from build123d import *

# Parameters (mm, degrees)
CYLINDER_R        = 1.3
CYLINDER_DEPTH    = 8
CYLINDER001_R     = 1.3
CYLINDER001_DEPTH = 8
EXTRUDE_DEPTH     = 15
CHAMFER_SIZE      = 2


with BuildPart() as cylinder000:
    # Cylinder → Cylinder (new body)
    with BuildSketch(Plane(origin=(12.5, -7.5, 0), x_dir=(1, 0, 0), z_dir=(0, 0, 1))):
        Circle(CYLINDER_R)
    extrude(amount=CYLINDER_DEPTH)


with BuildPart() as fusion:
    # Cylinder001 → Cylinder001 (new body)
    with BuildSketch(Plane(origin=(12.5, -7.5, 36), x_dir=(1, 0, 0), z_dir=(0, 0, 1))):
        Circle(CYLINDER001_R)
    extrude(amount=CYLINDER001_DEPTH)

    # Fusion: union Cylinder000
    add(cylinder000.part)


with BuildPart() as cut:
    # Sketch → Extrude (new body)
    with BuildSketch(Plane.XZ):
        Polygon((0, 0), (25, 0), (10, 15), (10, 29), (25, 44), (0, 44), align=None)
    extrude(amount=EXTRUDE_DEPTH)

    # Chamfer
    chamfer_edges = [cut.edges().sort_by_distance(p)[0] for p in [
        (0, 0, 22),
        (0, -15, 22),
        (17.5, 0, 7.5),
        (17.5, -15, 7.5),
        (10, 0, 22),
        (10, -15, 22),
        (17.5, 0, 36.5),
        (17.5, -15, 36.5),
    ]]
    chamfer(chamfer_edges, length=CHAMFER_SIZE)

    # Cut: cut Fusion
    add(fusion.part, mode=Mode.SUBTRACT)


solid = cut.part
Check sheet for the modelled part. Datum: model origin and axes. Units: mm. A direction names the side the tool comes from. Round coordinates to 2 decimals unless told otherwise and drop trailing zeros. Order: outer loops, then holes, each group sorted by start corner. A loop starts at its lowest first (then second) coordinate and runs counter-clockwise, first axis right, second up. Notation, with made-up numbers: M 36.25,23 L 67.25,23 A25 ccw 67.25,62 Z; hole C -26.75,2 d6. An arc over 180 degrees is marked long. One line per item, written item: value. Start each with the question number.
1. Section check C-C on y = -7.5. Enter the section's corners in (x, z), and give its area (3 significant figures).
2. Access from +Z, -Z, +X, -X, +Y, -Y to the whole of each face (thin tool, end or side, straight path). Record for faces 5 (the flat face through (18, -7, 7)), 6 (the flat face through (9, -1, 22)), 7 (the cylindrical face through (12.22, -8.77, 3.94)), 8 (the flat face through (16.381, -14.014, 36.815)), 9 (the cylindrical face through (12.22, -8.77, 39.94)).
3. Release check for a two-part mould opening along Z. For faces 1 (the flat face through (16.6, -0.99, 6.97)), 2 (the flat face through (16.381, -0.986, 36.815)), 3 (the flat face through (12, -7, 36)), 4 (the flat face through (1, -1, 22)) record: released by +Z, released by -Z, zero draft, split by the parting line, or undercut.
4. Section check A-A on x = 12.5. Enter the section's corners in (y, z).
5. Section check B-B on z = 21. Enter the section's corners in (x, y), and give its area (3 significant figures).
6. Scan lines: line 1 along Y through (x, z) = (12.5, 39.25); line 2 along Z through (x, y) = (17, -10.25); line 3 along Z through (x, y) = (18.5, -10.5). Record each from-to range of solid material in increasing order.
7. Section check D-D on z = 7. Enter the section's corners in (x, y).
8. Gauge pin test, flat ends, axial feed: P1, Ø9, axis at y = -8, z = 21.5, coming from the +X side; P2, Ø2, axis at x = 12.5, y = -7.5, coming from the +Z side; P3, Ø6, axis at y = -12.5, z = 15, coming from the +X side. Record the tip position at first contact, or that the pin passes through.
Results found:
1. outline: M 0,0 L 11.2,0 L 11.2,8 L 13.8,8 L 13.8,0 L 25,0 L 10,15 L 10,29 L 25,44 L 13.8,44 L 13.8,36 L 11.2,36 L 11.2,44 L 0,44 Z
1. area: 623 mm^2
2. face 5: +X, +Y, -Y
2. face 6: +X, +Y
2. face 7: -Z
2. face 8: +X, -Y
2. face 9: +Z
3. face 1: undercut
3. face 2: undercut
3. face 3: released by +Z
3. face 4: zero draft
4. outline: M -15,0 L -8.8,0 L -8.8,8 L -6.2,8 L -6.2,0 L 0,0 L 0,9.67 L -2,12.5 L -13,12.5 L -15,9.67 Z; M -15,34.33 L -13,31.5 L -2,31.5 L 0,34.33 L 0,44 L -6.2,44 L -6.2,36 L -8.8,36 L -8.8,44 L -15,44 Z
5. outline: M 0,-13 L 2,-15 L 8,-15 L 10,-13 L 10,-2 L 8,0 L 2,0 L 0,-2 Z
5. area: 142 mm^2
6. line 1: -15 to -8.8, -6.2 to 0
6. line 2: 0 to 8, 36 to 44
6. line 3: 0 to 6.5, 37.5 to 44
7. outline: M 0,-13 L 2,-15 L 15.17,-15 L 18,-13 L 18,-2 L 15.17,0 L 2,0 L 0,-2 Z; hole C 12.5,-7.5 d2.6
8. P1: x = 10
8. P2: z = 36
8. P3: x = 13
